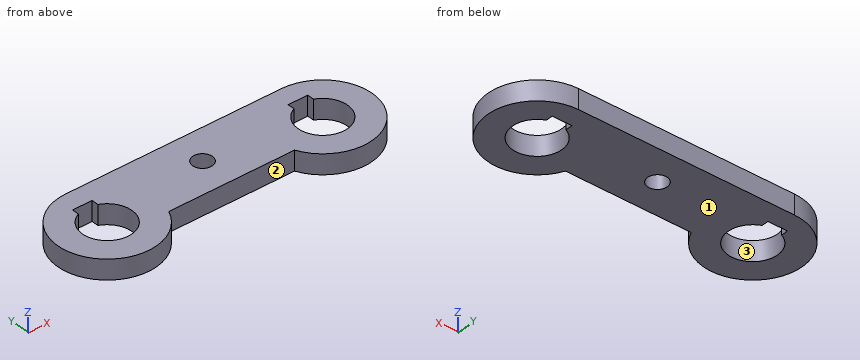
```python
from build123d import *

# Parameters (mm, degrees)
SKETCH_R     = 1
SKETCH_R_2   = 2.5
PAD_DEPTH    = 2
SKETCH001_W  = 2
SKETCH001_H  = 2
POCKET_DEPTH = 2.001


with BuildPart() as part:
    # Sketch → Pad (new body)
    with BuildSketch(Plane.XY):
        with BuildLine():
            Line((-11, 3.5), (11, 3.5))
            ThreePointArc((6.417424, -3.5), (15.1833, -4.238613), (11, 3.5))
            Line((-6.417424, -3.5), (6.417424, -3.5))
            ThreePointArc((-11, 3.5), (-15.1833, -4.238613), (-6.417424, -3.5))
        make_face()
        Circle(SKETCH_R, mode=Mode.SUBTRACT)
        with Locations((-11, -1.5)):
            Circle(SKETCH_R_2, mode=Mode.SUBTRACT)
        with Locations((11, -1.5)):
            Circle(SKETCH_R_2, mode=Mode.SUBTRACT)
    extrude(amount=PAD_DEPTH)

    # Sketch001 → Pocket (cut, through all)
    with BuildSketch(Plane.XY.offset(2)):
        with Locations((-11, 0.5)):
            Rectangle(SKETCH001_W, SKETCH001_H)
        with Locations((11, 0.5)):
            Rectangle(SKETCH001_W, SKETCH001_H)
    extrude(amount=-POCKET_DEPTH, mode=Mode.SUBTRACT)


solid = part.part
```
Source: CAD feature listing. Evaluate the final solid. Frame: model axes, mm. Face numbers are marked on the shaded views. Give positions to 0.01 mm unless a question says otherwise; leave off trailing zeros. Loops run counter-clockwise (first coordinate to the right, second up) from the corner with the lowest first, then second, coordinate; pieces in that order, holes last. Notation, with made-up numbers: (76, -5.5) - (112, -5.5) arc R19 ccw to (112, 16.5) - close; hole circle Ø6 at (20, 54.5). An arc over 180 degrees is marked (long way). Use CSV: the item, a comma, the result in double quotes. Start each with the question number.
1. Pin query (flat end, axial travel): pin 1 (0.6 mm diameter, centred on x = 1, z = 1, fed in from -Y); pin 2 (0.8 mm diameter, centred on y = 1, z = 1, fed in from +X); pin 3 (0.6 mm diameter, centred on y = 1, z = 0.5, fed in from -X). Return the tip coordinate at first contact, or that it passes through.
2. Section C-C (z = 1.65). Output: boundary loops of the cut face in (x, y).
3. Draft query along Y for the marked faces 1, 2 and 3. Return one class per face: +Y half, -Y half, draft (parallel to the pull), parting line (faces both ways), or undercut.
4. Section B-B (x = 0). Output: boundary loops of the cut face in (y, z), then the cut area to 3 significant figures.
5. Section A-A (y = -4.5). Output: boundary loops of the cut face in (x, z), then the cut area to 3 significant figures.
6. Ray query, L1, parallel to X at y = -1.5, z = 1.45; L2, parallel to X at y = 0.5, z = 1.05; L3, parallel to Y at x = -11, z = 0.55. Return the intervals inside material, ascending.
7. Section D-D (y = -1.5). Output: boundary loops of the cut face in (x, z).
Response:
1,pin 1,"y = -3.5"
1,pin 2,"x = 15.54"
1,pin 3,"x = -15.49"
2,outline,"(-11, 3.5) arc R5 ccw (long way) to (-6.42, -3.5) - (6.42, -3.5) arc R5 ccw (long way) to (11, 3.5) - close; hole (-12, 0.79) arc R2.5 ccw (long way) to (-10, 0.79) - (-10, 1.5) - (-12, 1.5) - close; hole circle Ø2 at (0, 0); hole (10, 0.79) arc R2.5 ccw (long way) to (12, 0.79) - (12, 1.5) - (10, 1.5) - close"
3,face 1,"draft"
3,face 2,"-Y half"
3,face 3,"undercut"
4,outline,"(-3.5, 0) - (-1, 0) - (-1, 2) - (-3.5, 2) - close; (1, 0) - (3.5, 0) - (3.5, 2) - (1, 2) - close"
4,area,"10.0 mm²"
5,outline,"(-15, 0) - (-7, 0) - (-7, 2) - (-15, 2) - close; (7, 0) - (15, 0) - (15, 2) - (7, 2) - close"
5,area,"32.0 mm²"
6,L1,"-16 to -13.5, -8.5 to 8.5, 13.5 to 16"
6,L2,"-15.58 to -12.5, -9.5 to -0.87, 0.87 to 9.5, 12.5 to 15.58"
6,L3,"-6.5 to -4, 1.5 to 3.5"
7,outline,"(-16, 0) - (-13.5, 0) - (-13.5, 2) - (-16, 2) - close; (-8.5, 0) - (8.5, 0) - (8.5, 2) - (-8.5, 2) - close; (13.5, 0) - (16, 0) - (16, 2) - (13.5, 2) - close"
